For this review, take the finished solid that the model builds, in its own axes (mm). A direction names the side the tool comes from. Coordinates: 2 decimals unless noted, no trailing zeros. Order: outer loops, then holes, each group sorted by start corner. A loop starts at its lowest first (then second) coordinate and runs counter-clockwise, first axis right, second up. Notation, with made-up numbers: (45, 79.25) -> (62, 79.25) arc R19 cw to (62, 115.25) -> close; hole circle Ø5 at (16, -12.75). An arc over 180 degrees is marked (long way). Answer as a JSON object with one key per item and string values. Group by question number.
1) Add section D-D, the plane y = 25.5. Write out the cut boundary in (x, z) (3 decimals), then the cut area to 3 significant figures.
2) Add section B-B, the plane z = 7.62. Write out the cut boundary in (x, y) (3 decimals).
3) Draft analysis for pull direction Y (two halves, no side actions). For faces 1 (the flat face through (-17.78, 24, -80)), 2 (the flat face through (-3, 48.26, -63)), 3 (the flat face through (-16, 43.18, -29)), 4 (the cylindrical face through (-1.6, 41.4, -134.1)), state which applies: +Y half, -Y half, draft (parallel to the pull), parting line (faces both ways), or undercut.
4) For pin 1 (8 mm diameter, centred on x = -8, z = -25, fed in from +Y); pin 2 (3.5 mm diameter, centred on x = -16.5, y = 18.5, fed in from +Z); pin 3 (4 mm diameter, centred on y = 20, z = -14, fed in from -X) (3 decimals), all flat-tipped, find the tip position at first contact; note any pin that passes through.
5) Wall thickness on L1, parallel to Z at x = -1.35, y = 40.64 (3 decimals); L2, parallel to Y at x = -1.15, z = 7.62; L3, parallel to X at y = 7, z = -101 (3 decimals): over which ranges is each line inside the solid? List them lowest first.
6) Add section A-A, the plane y = 7.62. Write out the cut boundary in (x, z) (3 decimals), then the cut area to 3 significant figures.
7) Machinability: for faces 5 (the flat face through (-14.605, 27, -93)), 6 (the flat face through (-16, 24, -53.975)), 7 (the flat face through (-3.175, 24, 8)), which of the approach directions +Z, -Z, +X, -X, +Y, -Y give a long, thin tool a straight path to every point of the face, cutting with its end or side? Answer none if there is none.
8) Add section C-C, the plane x = -6.5. Write out the cut boundary in (y, z) (3 decimals), then the cut area to 3 significant figures.
Autodesk Inventor part; units mm, degrees
ref_plane "YZ Plane" through (0, 0, 0) normal (1, 0, 0) x (0, 1, 0)
ref_plane "XZ Plane" through (0, 0, 0) normal (0, 1, 0) x (-1, 0, 0)
ref_plane "XY Plane" through (0, 0, 0) normal (0, 0, 1) x (1, 0, 0)
sketch "Sketch1" plane through (0, 0, 0) normal (0, 1, 0) x (-1, 0, 0)
  line L0 (0, 0) -> (0, -128.905)
  line L1 (0, -128.905) -> (17.78, -128.905)
  line L2 (17.78, -128.905) -> (17.78, 0)
  line L3 (17.78, 0) -> (0, 0)
  dimension "d0" = 128.905
  dimension "d1" = 17.78
extrude "Extrusion1" add sketch "Sketch1" along normal blind 48.26
sketch "Sketch2" plane through (0, 48.26, 0) normal (0, 1, 0) x (1, 0, 0)
  line L0 (0, 0) -> (0, 3.175)
  line L1 (0, 0) -> (0, 128.905)
  line L2 (0, 3.175) -> (-3.175, 3.175)
  line L3 (-3.175, 3.175) -> (-3.175, 125.73)
  line L4 (-3.175, 125.73) -> (-14.605, 125.73)
  line L5 (-14.605, 125.73) -> (-14.605, 3.175)
  line L6 (-14.605, 3.175) -> (-3.175, 3.175)
  dimension "d4" = 3.175
  dimension "d5" = 3.175
  dimension "d6" = 122.555
  dimension "d7" = 11.43
extrude "Extrusion2" cut sketch "Sketch2" against normal blind 43.18
sketch "Sketch3" plane through (-17.78, 0, -128.905) normal (-1, 0, 0) x (0, 0, 1)
  line L0 (128.905, 0) -> (125.73, 0)
  line L1 (128.905, 0) -> (0, 0)
  line L2 (125.73, 0) -> (125.73, 5.08)
  line L3 (125.73, 5.08) -> (74.93, 5.08)
  line L4 (3.175, 5.08) -> (125.73, 5.08)
  line L5 (74.93, 5.08) -> (74.93, 43.18)
  line L6 (0, 48.26) -> (128.905, 48.26)
  line L7 (74.93, 43.18) -> (125.73, 43.18)
  line L8 (125.73, 48.26) -> (125.73, 5.08)
  dimension "d10" = 3.175
  dimension "d11" = 5.08
  dimension "d12" = 50.8
  dimension "d13" = 38.1
extrude "Extrusion3" cut sketch "Sketch3" against normal blind 5.08
sketch "Sketch4" plane through (-17.78, 0, 0) normal (0, 0, 1) x (1, 0, 0)
  line L0 (17.78, 0) -> (14.605, 0)
  line L1 (0, 0) -> (17.78, 0)
  line L2 (14.605, 0) -> (14.605, 48.26)
  line L3 (17.78, 48.26) -> (0, 48.26)
  line L4 (17.78, 48.26) -> (17.78, 0)
  line L5 (17.78, 0) -> (17.78, 48.26)
  dimension "d16" = 3.175
extrude "Extrusion4" add sketch "Sketch4" along normal blind 15.24
sketch "Sketch5" plane through (-3.175, 0, 0) normal (-1, 0, 0) x (0, 0, 1)
  line L0 (15.24, 48.26) -> (7.62, 48.26)
  line L1 (0, 48.26) -> (15.24, 48.26)
  line L2 (7.62, 48.26) -> (7.62, 40.64)
  circle A0 centre (7.62, 40.64) radius 2.54
  line L3 (15.24, 0) -> (7.62, 0)
  line L4 (0, 0) -> (15.24, 0)
  line L5 (7.62, 0) -> (7.62, 7.62)
  circle A1 centre (7.62, 7.62) radius 2.54
  dimension "d19" = 7.62
  dimension "d20" = 7.62
  dimension "d21" = 5.08
  dimension "d22" = 7.62
  dimension "d23" = 7.62
  dimension "d24" = 5.08
extrude "Extrusion5" cut sketch "Sketch5" against normal blind 15.24
sketch "Sketch6" plane through (0, 0, -128.905) normal (0, 0, -1) x (-1, 0, 0)
  line L0 (0, 48.26) -> (3.175, 48.26)
  line L1 (3.175, 48.26) -> (3.175, 0)
  line L2 (3.175, 48.26) -> (3.175, 0)
  line L3 (3.175, 0) -> (0, 0)
  line L4 (0, 0) -> (0, 48.26)
  line L5 (0, 0) -> (0, 48.26)
  dimension "d27" = 3.175
extrude "Extrusion6" add sketch "Sketch6" along normal blind 15.24
sketch "Sketch7" plane through (-3.175, 0, -128.905) normal (-1, 0, 0) x (0, 0, 1)
  line L0 (-15.24, 48.26) -> (-15.24, 40.64)
  line L1 (-15.24, 48.26) -> (-15.24, 0)
  line L2 (-15.24, 40.64) -> (-7.62, 40.64)
  line L3 (-15.24, 0) -> (-7.62, 0)
  line L4 (0, 0) -> (-15.24, 0)
  line L5 (-7.62, 0) -> (-7.62, 7.62)
  circle A0 centre (-7.62, 7.62) radius 2.54
  circle A1 centre (-7.62, 40.64) radius 2.54
  point P0 (128.905, 0)
  dimension "d30" = 7.62
  dimension "d31" = 7.62
  dimension "d32" = 7.62
  dimension "d33" = 7.62
  dimension "d34" = 5.08
  dimension "d35" = 5.08
extrude "Extrusion7" cut sketch "Sketch7" against normal blind 15.24
properties part number "Autonomous - Phone Case V2"
Output values:
{
 "1": {"outline": "(-17.78, -128.905) -> (-3.175, -128.905) -> (-3.175, -144.145) -> (0, -144.145) -> (0, 15.24) -> (-3.175, 15.24) -> (-3.175, 0) -> (-17.78, 0) -> (-17.78, -3.175) -> (-3.175, -3.175) -> (-3.175, -125.73) -> (-14.605, -125.73) -> (-14.605, -53.975) -> (-17.78, -53.975) -> close", "area": "827 mm²"},
 "2": {"outline": "(-3.175, 0) -> (0, 0) -> (0, 5.08) -> (-3.175, 5.08) -> close; (-3.175, 10.16) -> (0, 10.16) -> (0, 38.1) -> (-3.175, 38.1) -> close; (-3.175, 43.18) -> (0, 43.18) -> (0, 48.26) -> (-3.175, 48.26) -> close"},
 "3": {"face 1": "draft", "face 2": "+Y half", "face 3": "undercut", "face 4": "undercut"},
 "4": {"pin 1": "stops at y = 5.08", "pin 2": "stops at z = 0", "pin 3": "stops at x = -3.175"},
 "5": {"L1": "z = -144.145 to -139.065, -133.985 to 5.08, 10.16 to 15.24", "L2": "y = 0 to 5.08, 10.16 to 38.1, 43.18 to 48.26", "L3": "x = -17.78 to -14.605, -3.175 to 0"},
 "6": {"outline": "(-17.78, -128.905) -> (-3.175, -128.905) -> (-3.175, -133.985) -> (0, -133.985) -> (0, 5.08) -> (-3.175, 5.08) -> (-3.175, 0) -> (-17.78, 0) -> (-17.78, -3.175) -> (-3.175, -3.175) -> (-3.175, -125.73) -> (-14.605, -125.73) -> (-14.605, -53.975) -> (-17.78, -53.975) -> close; (-3.175, -144.145) -> (0, -144.145) -> (0, -139.065) -> (-3.175, -139.065) -> close; (-3.175, 10.16) -> (0, 10.16) -> (0, 15.24) -> (-3.175, 15.24) -> close", "area": "794 mm²"},
 "7": {"face 5": "+Y", "face 6": "-X", "face 7": "+Z, -X, +Y, -Y"},
 "8": {"outline": "(0, -128.905) -> (48.26, -128.905) -> (48.26, -125.73) -> (5.08, -125.73) -> (5.08, -3.175) -> (48.26, -3.175) -> (48.26, 0) -> (0, 0) -> close", "area": "929 mm²"}
}
